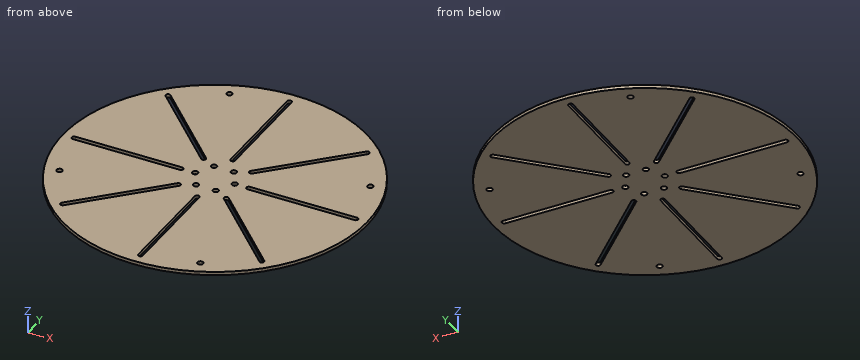
```python
from build123d import *

# Parameters (mm, degrees)
SKETCH1_R           = 135
SKETCH1_R_2         = 2.5
BOSS_EXTRUDE1_DEPTH = 3


with BuildPart() as part:
    # Sketch1 → Boss-Extrude1 (new body)
    with BuildSketch(Plane.XY):
        Circle(SKETCH1_R)
        with Locations((-17.5, 0)):
            Circle(SKETCH1_R_2, mode=Mode.SUBTRACT)
        with Locations((-46.878720465, 113.175242733)):
            Circle(SKETCH1_R_2, mode=Mode.SUBTRACT)
        with Locations((113.175242733, 46.878720465)):
            Circle(SKETCH1_R_2, mode=Mode.SUBTRACT)
        with Locations((46.878720465, -113.175242733)):
            Circle(SKETCH1_R_2, mode=Mode.SUBTRACT)
        with Locations((-8.75, 15.155444566)):
            Circle(SKETCH1_R_2, mode=Mode.SUBTRACT)
        with Locations((8.75, 15.155444566)):
            Circle(SKETCH1_R_2, mode=Mode.SUBTRACT)
        with Locations((17.5, 0)):
            Circle(SKETCH1_R_2, mode=Mode.SUBTRACT)
        with Locations((8.75, -15.155444566)):
            Circle(SKETCH1_R_2, mode=Mode.SUBTRACT)
        with Locations((-8.75, -15.155444566)):
            Circle(SKETCH1_R_2, mode=Mode.SUBTRACT)
        with Locations((-113.175242733, -46.878720465)):
            Circle(SKETCH1_R_2, mode=Mode.SUBTRACT)
        with BuildLine():
            Line((30, 2), (125, 2))
            ThreePointArc((125, 2), (127, 0), (125, -2))
            Line((125, -2), (30, -2))
            ThreePointArc((30, -2), (28, 0), (30, 2))
        make_face(mode=Mode.SUBTRACT)
        with BuildLine():
            Line((22.627416998, -19.798989873), (89.802561211, -86.974134086))
            ThreePointArc((89.802561211, -86.974134086), (89.802561211, -89.802561211), (86.974134086, -89.802561211))
            Line((86.974134086, -89.802561211), (19.798989873, -22.627416998))
            ThreePointArc((19.798989873, -22.627416998), (19.798989873, -19.798989873), (22.627416998, -19.798989873))
        make_face(mode=Mode.SUBTRACT)
        with BuildLine():
            Line((2, -30), (2, -125))
            ThreePointArc((2, -125), (0, -127), (-2, -125))
            Line((-2, -125), (-2, -30))
            ThreePointArc((-2, -30), (0, -28), (2, -30))
        make_face(mode=Mode.SUBTRACT)
        with BuildLine():
            Line((-19.798989873, -22.627416998), (-86.974134086, -89.802561211))
            ThreePointArc((-86.974134086, -89.802561211), (-89.802561211, -89.802561211), (-89.802561211, -86.974134086))
            Line((-89.802561211, -86.974134086), (-22.627416998, -19.798989873))
            ThreePointArc((-22.627416998, -19.798989873), (-19.798989873, -19.798989873), (-19.798989873, -22.627416998))
        make_face(mode=Mode.SUBTRACT)
        with BuildLine():
            Line((-30, -2), (-125, -2))
            ThreePointArc((-125, -2), (-127, 0), (-125, 2))
            Line((-125, 2), (-30, 2))
            ThreePointArc((-30, 2), (-28, 0), (-30, -2))
        make_face(mode=Mode.SUBTRACT)
        with BuildLine():
            Line((-22.627416998, 19.798989873), (-89.802561211, 86.974134086))
            ThreePointArc((-89.802561211, 86.974134086), (-89.802561211, 89.802561211), (-86.974134086, 89.802561211))
            Line((-86.974134086, 89.802561211), (-19.798989873, 22.627416998))
            ThreePointArc((-19.798989873, 22.627416998), (-19.798989873, 19.798989873), (-22.627416998, 19.798989873))
        make_face(mode=Mode.SUBTRACT)
        with BuildLine():
            Line((-2, 30), (-2, 125))
            ThreePointArc((-2, 125), (0, 127), (2, 125))
            Line((2, 125), (2, 30))
            ThreePointArc((2, 30), (0, 28), (-2, 30))
        make_face(mode=Mode.SUBTRACT)
        with BuildLine():
            Line((19.798989873, 22.627416998), (86.974134086, 89.802561211))
            ThreePointArc((86.974134086, 89.802561211), (89.802561211, 89.802561211), (89.802561211, 86.974134086))
            Line((89.802561211, 86.974134086), (22.627416998, 19.798989873))
            ThreePointArc((22.627416998, 19.798989873), (19.798989873, 19.798989873), (19.798989873, 22.627416998))
        make_face(mode=Mode.SUBTRACT)
    extrude(amount=BOSS_EXTRUDE1_DEPTH)


solid = part.part
```
Build history of the part. All positions in model axes, mm. Round coordinates to 2 decimals unless told otherwise and drop trailing zeros. Write each loop counter-clockwise with the first axis right and the second up, starting at its lowest first coordinate (ties: lowest second). Pieces come first, ordered by that corner, then holes. Notation, with made-up numbers: (-7, -27) -> (5, -27) arc R20 cw to (5, 4) -> close; hole circle Ø10 at (-35, -9). An arc over 180 degrees is marked (long way). Put each result on its own line as item: value.
Item 1: Slice it at A-A, the plane y = 73. Give the cut face in (x, z), plus the area to 3 significant figures.
Here are the results:
outline: (-113.56, 0) -> (-75.83, 0) -> (-75.83, 3) -> (-113.56, 3) -> close; (-70.17, 0) -> (-2, 0) -> (-2, 3) -> (-70.17, 3) -> close; (2, 0) -> (70.17, 0) -> (70.17, 3) -> (2, 3) -> close; (75.83, 0) -> (113.56, 0) -> (113.56, 3) -> (75.83, 3) -> close
area: 635 mm^2
Item 2: Flat gauge pins, fed straight in: P1, Ø10, axis at x = -6, y = 77.5, coming from the -Z side; P2, Ø1.5, axis at y = -79.5, z = 2, coming from the +X side; P3, Ø1.5, axis at x = 77.5, z = 1, coming from the -Y side; P4, Ø1.5, axis at x = 73, z = 1.5, coming from the +Y side. Where does each tip first touch, or does it go through?
Here are the results:
P1: stops at z = 0
P2: stops at x = 109.65
P3: stops at y = -111.06
P4: stops at y = 114.04
Item 3: Slice it at C-C, the plane z = 0.5. Count the separate pieces of the cut face and the enclosed holes in it, plus the area to 3 significant figures.
Here are the results:
separate pieces: 1
enclosed holes: 18
area: 53,900 mm^2
Item 4: Wall check: probe 1 along Y at (x, z) = (-19.5, 2.75); probe 2 along Y at (x, z) = (-45.5, 1.15); probe 3 along Y at (x, z) = (-48, 2.35). Give the ranges that are in metal, low to high. Write a range as from..to.
Here are the results:
probe 1: y = -133.58..-22.25, -20.18..-1.5, 1.5..20.18, 22.25..133.58
probe 2: y = -127.1..-48.33, -42.67..-2, 2..42.67, 48.33..111.09, 115.26..127.1
probe 3: y = -126.18..-50.83, -45.17..-2, 2..45.17, 50.83..110.94, 115.41..126.18
Item 5: Slice it at B-B, the plane x = 80. Give the cut face in (y, z), plus the area to 3 significant figures.
Here are the results:
outline: (-108.74, 0) -> (-82.83, 0) -> (-82.83, 3) -> (-108.74, 3) -> close; (-77.17, 0) -> (-2, 0) -> (-2, 3) -> (-77.17, 3) -> close; (2, 0) -> (77.17, 0) -> (77.17, 3) -> (2, 3) -> close; (82.83, 0) -> (108.74, 0) -> (108.74, 3) -> (82.83, 3) -> close
area: 607 mm^2
